CAD build for the part. Positions are in the model's coordinates, mm. A direction names the side the tool comes from. Give positions to 0.01 mm unless a question says otherwise; leave off trailing zeros. Loops run counter-clockwise (first coordinate to the right, second up) from the corner with the lowest first, then second, coordinate; pieces in that order, holes last. Notation, with made-up numbers: (49.5, -24) -> (94.5, -24) arc R21 ccw to (94.5, -2) -> close; hole circle Ø2 at (37.5, -33.5). An arc over 180 degrees is marked (long way). Use one line per item in the form item = value.
```python
from build123d import *

# Parameters (mm, degrees)
SKETCH1_W   = 10.5
SKETCH1_H   = 14.5
SKETCH1_W_2 = 11
SKETCH1_H_2 = 7.5


with BuildPart() as part:
    # Sketch1 → Revolve1 (revolve)
    with BuildSketch(Plane(origin=(0, 0, 0), x_dir=(0, 0, -1), z_dir=(1, 0, 0)), mode=Mode.PRIVATE) as revolve1_sk:
        with Locations((5.25, 7.25)):
            Rectangle(SKETCH1_W, SKETCH1_H)
        Polygon((10.5, 14.5), (10.5, 0), (22, 0), (22, 18.25), (10.5, 18.25), align=None)
        Polygon((22, 18.25), (22, 0), (36, 0), (36, 16.5), (36, 21.5), (22, 21.5), align=None)
        Polygon((36, 16.5), (36, 0), (45.5, 0), (45.5, 11.25), (45.5, 16.5), align=None)
        Polygon((45.5, 11.25), (45.5, 0), (57.5, 0), (57.5, 7.5), (57.5, 11.25), align=None)
        with Locations((63, 3.75)):
            Rectangle(SKETCH1_W_2, SKETCH1_H_2)
    revolve(revolve1_sk.sketch.rotate(Axis((0, 0, -22), (0, 0, -1)), 90), axis=Axis((0, 0, -22), (0, 0, -1)))


solid = part.part
```
1. Cut at C-C, the plane z = -51. Write the cut outline in (x, y), then the cut area to 3 significant figures.
Result sheet:
outline = circle Ø22.5 at (0, 0)
area = 398 mm^2
2. Drill centre lines: line 1 (Z direction, x = -5.5, y = -16); line 2 (Z direction, x = 11, y = -15); line 3 (Y direction, x = 3, z = -3). Where is each one in solid material? Low to high.
Result sheet:
line_1 = -36 to -10.5
line_2 = -36 to -22
line_3 = -14.19 to 14.19
3. Tool access for faces 1 (the flat face through (0, 0, 0)), 2 (the flat face through (-10, 16, -22)), 3 (the cylindrical face through (4.032, -6.324, -63.077)): list every direction of +Z, -Z, +X, -X, +Y, -Y with a clear straight run to the whole face (end or side of a thin tool).
Result sheet:
face_1 = +Z, +X, -X, +Y, -Y
face_2 = +Z
face_3 = -Z
4. Cut at A-A, the plane x = 0. Write the cut outline in (y, z).
Result sheet:
outline = (-21.5, -36) -> (-16.5, -36) -> (-16.5, -45.5) -> (-11.25, -45.5) -> (-11.25, -57.5) -> (-7.5, -57.5) -> (-7.5, -68.5) -> (7.5, -68.5) -> (7.5, -57.5) -> (11.25, -57.5) -> (11.25, -45.5) -> (16.5, -45.5) -> (16.5, -36) -> (21.5, -36) -> (21.5, -22) -> (18.25, -22) -> (18.25, -10.5) -> (14.5, -10.5) -> (14.5, 0) -> (-14.5, 0) -> (-14.5, -10.5) -> (-18.25, -10.5) -> (-18.25, -22) -> (-21.5, -22) -> close
5. Drop flat-ended pins along their axis: P1, Ø3, axis at y = 8.5, z = -16, coming from the +X side; P2, Ø3, axis at y = 3, z = -17.5, coming from the -X side; P3, Ø1, axis at x = -6.5, z = -48, coming from the -Y side. Give the stop position or say it passes through.
Result sheet:
P1 = 16.85
P2 = -18.19
P3 = -9.52
6. Cut at D-D, the plane x = -9. Write the cut outline in (y, z), then the cut area to 3 significant figures.
Result sheet:
outline = (-19.53, -36) -> (-13.83, -36) -> (-13.83, -45.5) -> (-6.75, -45.5) -> (-6.75, -57.5) -> (6.75, -57.5) -> (6.75, -45.5) -> (13.83, -45.5) -> (13.83, -36) -> (19.53, -36) -> (19.53, -22) -> (15.88, -22) -> (15.88, -10.5) -> (11.37, -10.5) -> (11.37, 0) -> (-11.37, 0) -> (-11.37, -10.5) -> (-15.88, -10.5) -> (-15.88, -22) -> (-19.53, -22) -> close
area = 1,580 mm^2
